Read the model definition and answer for the solid it produces. Units are mm, in the model's axes. Coordinates: 2 decimals unless noted, no trailing zeros. Order: outer loops, then holes, each group sorted by start corner. A loop starts at its lowest first (then second) coordinate and runs counter-clockwise, first axis right, second up. Notation, with made-up numbers: (20, 62) - (30, 62) arc R12 ccw to (30, 72) - close; hole circle Ø4 at (47.5, 53.5). An arc over 180 degrees is marked (long way). Use one line per item in the form item = value.
Autodesk Inventor part; units mm, degrees
ref_plane "YZ Plane" through (0, 0, 0) normal (1, 0, 0) x (0, 1, 0)
ref_plane "XZ Plane" through (0, 0, 0) normal (0, 1, 0) x (-1, 0, 0)
ref_plane "XY Plane" through (0, 0, 0) normal (0, 0, 1) x (1, 0, 0)
sketch "Sketch1" plane through (0, 0, 0) normal (0, 1, 0) x (-1, 0, 0)
  line L0 (0, 0) -> (-50, 0)
  line L1 (-50, 0) -> (-50, -15)
  line L2 (-50, -15) -> (0, -15)
  line L3 (0, -15) -> (0, 0)
  dimension "d0" = 50
  dimension "d1" = 15
extrude "Extrusion1" add sketch "Sketch1" along normal blind 1.6
sketch "Sketch2" plane through (0, 0, 0) normal (0, -1, 0) x (1, 0, 0)
  circle A0 centre (7.5, -7.5) radius 2
  line L0 (0, -15) -> (0, 0)
  circle A1 centre (42.5, -7.5) radius 2
  line L1 (50, 0) -> (50, -15)
  point P0 (0, -7.5)
  point P1 (50, -7.5)
  dimension "d4" = 4
  dimension "d5" = 7.5
  dimension "d6" = 4
  dimension "d7" = 7.5
extrude "Extrusion2" cut sketch "Sketch2" against normal blind 10
properties part number "Latch Catch Piece" material "Steel"
(1) Section A-A, the plane x = 7.5 is taken. Write down the section's boundary in (y, z).
Answer list:
outline = (0, -15) - (1.6, -15) - (1.6, -9.5) - (0, -9.5) - close; (0, -5.5) - (1.6, -5.5) - (1.6, 0) - (0, 0) - close
(2) Section B-B, the plane z = -7.5 is taken. Write down the section's boundary in (x, y), then the cut area to 3 significant figures.
Answer list:
outline = (0, 0) - (5.5, 0) - (5.5, 1.6) - (0, 1.6) - close; (9.5, 0) - (40.5, 0) - (40.5, 1.6) - (9.5, 1.6) - close; (44.5, 0) - (50, 0) - (50, 1.6) - (44.5, 1.6) - close
area = 67.2 mm2
(3) Section C-C, the plane y = 0.4 is taken. Write down the section's boundary in (x, z).
Answer list:
outline = (0, -15) - (50, -15) - (50, 0) - (0, 0) - close; hole circle Ø4 at (7.5, -7.5); hole circle Ø4 at (42.5, -7.5)
(4) The mould has two halves that part along X. Classify faces 1 (the flat face through (0, 1, -8)), 2 (the flat face through (25, 1.6, -7)), 3 (the flat face through (50, 1, -7)), 4 (the cylindrical face through (41.026, 0.789, -6.148)): +X half, -X half, draft (parallel to the pull), parting line (faces both ways), or undercut.
Answer list:
face_1 = -X half
face_2 = draft
face_3 = +X half
face_4 = undercut
(5) Straight lines are drawn through the part: L1, parallel to Z at x = 7.5, y = 1.2; L2, parallel to X at y = 1.05, z = -7.25; L3, parallel to X at y = 1.45, z = -8.5. For each, find the intervals that lie inside material, in ascending order.
Answer list:
L1 = -15 to -9.5, -5.5 to 0
L2 = 0 to 5.52, 9.48 to 40.52, 44.48 to 50
L3 = 0 to 5.77, 9.23 to 40.77, 44.23 to 50
